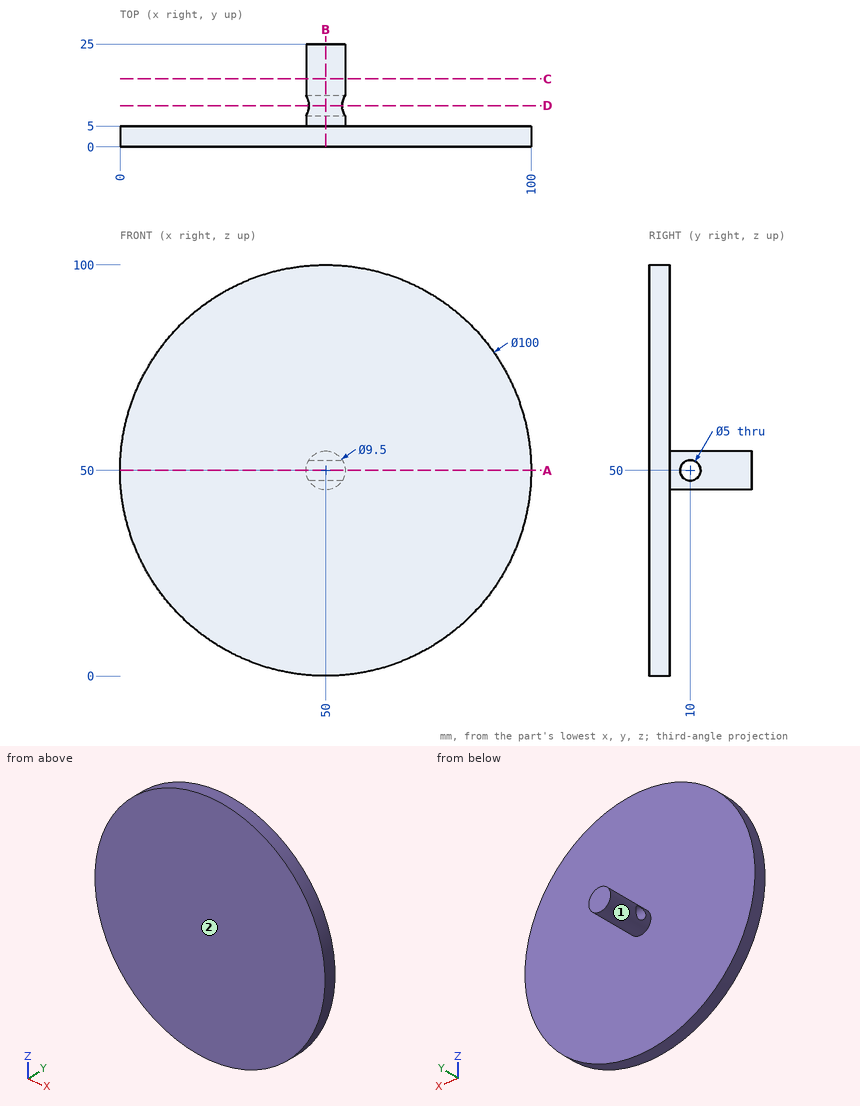
Geometry: see drawing. Coordinates: mm, zero at the bounding-box minimum. A direction names the side the tool comes from. Round coordinates to 2 decimals unless told otherwise and drop trailing zeros. Write each loop counter-clockwise with the first axis right and the second up, starting at its lowest first coordinate (ties: lowest second). Pieces come first, ordered by that corner, then holes. Notation, with made-up numbers: M 73.5,89 L 110.5,89 A14 ccw 110.5,110 Z; hole C -36,54.25 d1. An arc over 180 degrees is marked long. Answer as a JSON object with one key per item and string values. Group by question number.
(1) Section query A-A on z = 50. Output: boundary loops of the cut face in (x, y).
(2) First-contact query: pin 1 (2 mm diameter, centred on x = 49, z = 82, fed in from +Y); pin 2 (6 mm diameter, centred on y = 10, z = 50, fed in from -X); pin 3 (10 mm diameter, centred on x = 54.5, y = 8.5, fed in from -Z). Flat tips, straight axial feed; report the tip coordinate or a pass-through.
(3) Section query B-B on x = 50. Output: boundary loops of the cut face in (y, z), then the cut area to 3 significant figures.
(4) Ray query, line 1 (Y direction, x = 51.25, z = 50); line 2 (Z direction, x = 49.5, y = 10); line 3 (Y direction, x = 29, z = 65). Return the intervals inside material, ascending. Write a range as [from, to].
(5) Section query D-D on y = 10. Output: boundary loops of the cut face in (x, z).
(6) Section query C-C on y = 16.5. Output: boundary loops of the cut face in (x, z).
(7) Reachability of the marked faces 1 and 2 from +Z, -Z, +X, -X, +Y, -Y: full face, straight path, thin tool, end or side. Return the list, or none.
Computed values:
{
 "1": {"outline": "M 0,0 L 100,0 L 100,5 L 54.75,5 L 54.75,7.5 L 45.25,7.5 L 45.25,5 L 0,5 Z; M 45.25,12.5 L 54.75,12.5 L 54.75,25 L 45.25,25 Z"},
 "2": {"pin 1": "y = 5", "pin 2": "x = 45.25", "pin 3": "z = 0.01"},
 "3": {"outline": "M 0,0 L 5,0 L 5,45.25 L 25,45.25 L 25,54.75 L 5,54.75 L 5,100 L 0,100 Z; hole C 10,50 d5", "area": "670 mm^2"},
 "4": {"line 1": "[0, 7.5], [12.5, 25]", "line 2": "[45.28, 47.5], [52.5, 54.72]", "line 3": "[0, 5]"},
 "5": {"outline": "M 45.96,47.5 A4.75 ccw 54.04,47.5 Z; M 45.96,52.5 L 54.04,52.5 A4.75 ccw Z"},
 "6": {"outline": "C 50,50 d9.5"},
 "7": {"face 1": "+Y", "face 2": "+Z, -Z, +X, -X, -Y"}
}
